Source: CAD feature listing. Evaluate the final solid. Frame: model axes, mm. Give positions to 0.01 mm unless a question says otherwise; leave off trailing zeros. Order: outer loops, then holes, each group sorted by start corner. A loop starts at its lowest first (then second) coordinate and runs counter-clockwise, first axis right, second up. Notation, with made-up numbers: (-12, 25) - (20, 25) arc R13 ccw to (20, 30) - close; hole circle Ø7 at (-7.75, -22.75). An arc over 180 degrees is marked (long way). Use CSV: the item, a comma, the result in double quotes.
```python
from build123d import *

# Parameters (mm, degrees)
F1_DEPTH = 292.1
F3_DEPTH = 241.3
F4_W     = 203.2
F4_H     = 292.1
F5_DEPTH = 266.7


with BuildPart() as f1:
    # F0 (on Front) → F1 (new body)
    with BuildSketch(Plane.XZ):
        with BuildLine():
            Line((-169.3378070244, 253.4319378298), (-56.4459356748, 84.4773126099))
            ThreePointArc((-56.4459356748, 84.4773126099), (-52.23283881, 87.145226776), (-47.8939084615, 89.6032004578))
            Line((-47.8939084615, 89.6032004578), (-143.6817253846, 268.8096013734))
            ThreePointArc((-143.6817253846, 268.8096013734), (-156.6985164301, 261.4356803281), (-169.3378070244, 253.4319378298))
        make_face()
        with BuildLine():
            Line((-304.8, 0), (-101.6, 0))
            ThreePointArc((-101.6, 0), (-101.4776183504, 4.9852757117), (-101.1107682299, 9.9585414575))
            Line((-101.1107682299, 9.9585414575), (-303.3323046897, 29.8756243725))
            ThreePointArc((-303.3323046897, 29.8756243725), (-304.4328550513, 14.955827135), (-304.8, 0))
        make_face()
        with BuildLine():
            ThreePointArc((-101.1107682299, 9.9585414575), (-100.5003334124, 14.9078162047), (-99.647784489, 19.8211767168))
            Line((-99.647784489, 19.8211767168), (-298.9433534669, 59.4635301505))
            ThreePointArc((-298.9433534669, 59.4635301505), (-301.5010002373, 44.723448614), (-303.3323046897, 29.8756243725))
            Line((-303.3323046897, 29.8756243725), (-101.1107682299, 9.9585414575))
        make_face()
        with BuildLine():
            Line((-193.3630730131, 235.613586185), (-64.454357671, 78.5378620617))
            ThreePointArc((-64.454357671, 78.5378620617), (-60.5230493364, 81.6058851984), (-56.4459356748, 84.4773126099))
            Line((-56.4459356748, 84.4773126099), (-169.3378070244, 253.4319378298))
            ThreePointArc((-169.3378070244, 253.4319378298), (-181.5691480093, 244.8176555953), (-193.3630730131, 235.613586185))
        make_face()
        with BuildLine():
            Line((-303.3323046897, -29.8756243724), (-101.1107682299, -9.9585414575))
            ThreePointArc((-101.1107682299, -9.9585414575), (-101.4776183504, -4.9852757117), (-101.6, 0))
            Line((-101.6, 0), (-304.8, 0))
            ThreePointArc((-304.8, 0), (-304.4328550513, -14.955827135), (-303.3323046897, -29.8756243724))
        make_face()
        with BuildLine():
            Line((-215.5261469057, 215.5261469057), (-71.8420489686, 71.8420489686))
            ThreePointArc((-71.8420489686, 71.8420489686), (-68.2303898125, 75.2806343361), (-64.454357671, 78.5378620617))
            Line((-64.454357671, 78.5378620617), (-193.3630730131, 235.613586185))
            ThreePointArc((-193.3630730131, 235.613586185), (-204.6911694374, 225.8419030082), (-215.5261469057, 215.5261469057))
        make_face()
        with BuildLine():
            ThreePointArc((-99.647784489, -19.8211767168), (-100.5003334124, -14.9078162047), (-101.1107682299, -9.9585414575))
            Line((-101.1107682299, -9.9585414575), (-303.3323046897, -29.8756243724))
            ThreePointArc((-303.3323046897, -29.8756243724), (-301.5010002373, -44.723448614), (-298.9433534669, -59.4635301505))
            Line((-298.9433534669, -59.4635301505), (-99.647784489, -19.8211767168))
        make_face()
        with BuildLine():
            Line((-235.613586185, 193.3630730131), (-78.5378620617, 64.454357671))
            ThreePointArc((-78.5378620617, 64.454357671), (-75.2806343361, 68.2303898125), (-71.8420489686, 71.8420489686))
            Line((-71.8420489686, 71.8420489686), (-215.5261469057, 215.5261469057))
            ThreePointArc((-215.5261469057, 215.5261469057), (-225.8419030082, 204.6911694374), (-235.613586185, 193.3630730131))
        make_face()
        with BuildLine():
            Line((-291.6754143312, -88.4787696272), (-97.2251381104, -29.4929232091))
            ThreePointArc((-97.2251381104, -29.4929232091), (-98.5551753246, -24.6867862782), (-99.647784489, -19.8211767168))
            Line((-99.647784489, -19.8211767168), (-298.9433534669, -59.4635301505))
            ThreePointArc((-298.9433534669, -59.4635301505), (-295.6655259737, -74.0603588345), (-291.6754143312, -88.4787696272))
        make_face()
        with BuildLine():
            Line((-268.8096013734, 143.6817253846), (-89.6032004578, 47.8939084615))
            ThreePointArc((-89.6032004578, 47.8939084615), (-87.145226776, 52.23283881), (-84.4773126099, 56.4459356748))
            Line((-84.4773126099, 56.4459356748), (-253.4319378298, 169.3378070244))
            ThreePointArc((-253.4319378298, 169.3378070244), (-261.4356803281, 156.6985164301), (-268.8096013734, 143.6817253846))
        make_face()
        with BuildLine():
            Line((-281.5984815094, 116.6419101849), (-93.8661605031, 38.8806367283))
            ThreePointArc((-93.8661605031, 38.8806367283), (-91.8453121813, 43.4395974925), (-89.6032004578, 47.8939084615))
            Line((-89.6032004578, 47.8939084615), (-268.8096013734, 143.6817253846))
            ThreePointArc((-268.8096013734, 143.6817253846), (-275.535936544, 130.3187924776), (-281.5984815094, 116.6419101849))
        make_face()
        with BuildLine():
            ThreePointArc((-97.2251381104, 29.4929232091), (-95.6608770226, 34.2280091047), (-93.8661605031, 38.8806367283))
            Line((-93.8661605031, 38.8806367283), (-281.5984815094, 116.6419101849))
            ThreePointArc((-281.5984815094, 116.6419101849), (-286.9826310678, 102.6840273139), (-291.6754143312, 88.4787696272))
            Line((-291.6754143312, 88.4787696272), (-97.2251381104, 29.4929232091))
        make_face()
        with BuildLine():
            Line((-253.4319378298, 169.3378070244), (-84.4773126099, 56.4459356748))
            ThreePointArc((-84.4773126099, 56.4459356748), (-81.6058851984, 60.5230493364), (-78.5378620617, 64.454357671))
            Line((-78.5378620617, 64.454357671), (-235.613586185, 193.3630730131))
            ThreePointArc((-235.613586185, 193.3630730131), (-244.8176555953, 181.5691480093), (-253.4319378298, 169.3378070244))
        make_face()
        with BuildLine():
            Line((-298.9433534669, 59.4635301505), (-99.647784489, 19.8211767168))
            ThreePointArc((-99.647784489, 19.8211767168), (-98.5551753246, 24.6867862782), (-97.2251381104, 29.4929232091))
            Line((-97.2251381104, 29.4929232091), (-291.6754143312, 88.4787696272))
            ThreePointArc((-291.6754143312, 88.4787696272), (-295.6655259737, 74.0603588345), (-298.9433534669, 59.4635301505))
        make_face()
    extrude(amount=F1_DEPTH)

    # F3 (add): a face of the model
    f3_faces = [f1.faces().sort_by_distance(p)[0] for p in [
        (-95.787816923, -146.05, 179.2064009156),
    ]]
    extrude(f3_faces, amount=F3_DEPTH)

    # F4 (on face) → F5 (join)
    with BuildSketch(Plane(origin=(0, 0, 0), x_dir=(0.9569403357, 0, 0.2902846773), z_dir=(0.2902846773, 0, -0.9569403357))):
        with Locations((-203.2, 146.05)):
            Rectangle(F4_W, F4_H)
    extrude(amount=F5_DEPTH)


solid = f1.part
```
Item 1: Mould query, pull axis Z, two halves, no side actions, for faces 1 (the flat face through (-59.06, -144.01, -155.31)), 2 (the flat face through (-118.393, -148.095, -314.615)), 3 (the flat face through (-38.768, -144.005, 324.887)). Classes: released by +Z, released by -Z, zero draft, split by the parting line, or undercut.
Filled in:
face 1,"undercut"
face 2,"released by -Z"
face 3,"released by +Z"
Item 2: First-contact query: pin 1 (5 mm diameter, centred on y = -91.5, z = 197.5, fed in from +X); pin 2 (6 mm diameter, centred on x = 94.5, y = -113.5, fed in from -Z); pin 3 (2 mm diameter, centred on y = -156.5, z = 174, fed in from +X). Flat tips, straight axial feed; report the tip coordinate or a pass-through.
Filled in:
pin 1,"stops at x = 158.64"
pin 2,"stops at z = 164.11"
pin 3,"stops at x = 111.87"
Item 3: Section A-A on y = -221.5. Return the cut outline in (x, z), then the cut area to 3 significant figures.
Filled in:
outline,"(-291.68, -88.48) - (-214.26, -343.69) - (-19.81, -284.71) - (-97.23, -29.49) arc R101.6 cw to (-47.89, 89.6) - (164.91, 203.35) - (69.13, 382.56) - (-143.68, 268.81) arc R304.8 ccw to start"
area,"160,000 mm2"
Item 4: Section C-C on z = 99. Return the cut outline in (x, y).
Filled in:
outline,"(-288.27, -292.1) - (-30.31, -292.1) - (-30.31, 0) - (-288.27, 0) - close"
Item 5: Section B-B on x = 31.5. Return the cut outline in (y, z), then the cut area to 3 significant figures.
Filled in:
outline,"(-292.1, 132.04) - (0, 132.04) - (0, 362.45) - (-292.1, 362.45) - close"
area,"67,300 mm2"
Item 6: Material intervals for line 1 (X direction, y = -267.5, z = 1); line 2 (Z direction, x = 128.5, y = -172.5); line 3 (Z direction, x = -10, y = -141.5), sorted ascending. Write a range as from..to.
Filled in:
line 1,"x = -304.8..-101.6"
line 2,"z = 183.89..271.48"
line 3,"z = 109.86..340.26"
